Design review of the part built by this model. Coordinates are the model's own, in mm. Face numbers are marked on the shaded views. A direction names the side the tool comes from. Round coordinates to 2 decimals unless told otherwise and drop trailing zeros. Write each loop counter-clockwise with the first axis right and the second up, starting at its lowest first coordinate (ties: lowest second). Pieces come first, ordered by that corner, then holes. Notation, with made-up numbers: (28.25, -38) -> (51.25, -38) arc R14 ccw to (51.25, -16) -> close; hole circle Ø5 at (63.25, 36.25). An arc over 180 degrees is marked (long way). One line per question, with ' | ' between items. Start each with the question number.
1) For probe 1 along Y at (x, z) = (-24.13, -1.2); probe 2 along X at (y, z) = (5.5, 4); probe 3 along Y at (x, z) = (-8.89, -0.9), list the stretches that pass through material, from the lowest coordinate up.
2) For the marked faces 1, 2 and 3, list the 3-axis set-ups (+Z, -Z, +X, -X, +Y, -Y) from which the entire face can be reached by the end or side of a thin tool; tool diameter is ignored.
3) Consider section A-A (z = 2). Give the boundary of the cut face in (x, y).
4) Consider section D-D (x = -24.13). Give the boundary of the cut face in (y, z).
5) Mouldability with a two-part tool opening along X and no side actions: class the marked faces 4, 5, 6 and 7 as +X half, -X half, draft (parallel to the pull), parting line (faces both ways), or undercut.
6) Consider section C-C (y = -15.5). Give the boundary of the cut face in (x, z).
7) Consider section B-B (x = -8.89). Give the boundary of the cut face in (y, z), then the cut area to 3 significant figures.
8) Insertion check: pin 1 Ø3 at (y, z) = (24, 2.5) entering from +X; pin 2 Ø1.3 at (x, z) = (-23.5, 4) entering from -Y; pin 3 Ø0.8 at (x, z) = (-23.5, 6.5) entering from +Y; pin 4 Ø3 at (x, y) = (-24.13, -19.05) entering from +Z. Each pin has a flat end and moves straight along its axis. Give the tip position at first contact, or say it passes through.
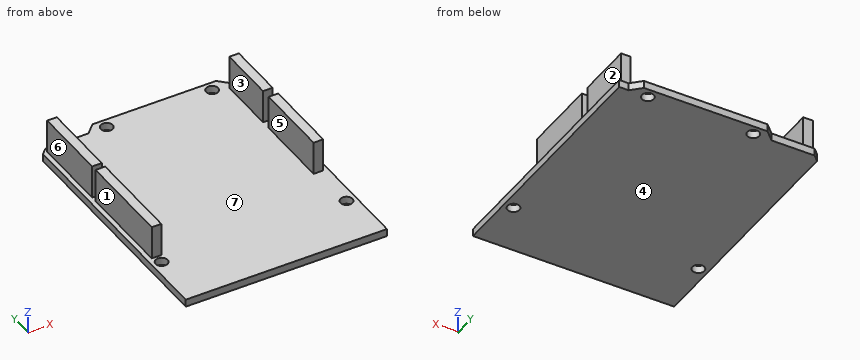
```python
from build123d import *

# Parameters (mm, degrees)
F0_W     = 53.34
F0_H     = 68.58
F1_DEPTH = 2
F3_DEPTH = 2
F6_D     = 3.175
F7_W     = 2.54
F7_H     = 20.32
F7_H_2   = 25.4
F7_H_3   = 15.24
F8_DEPTH = 8.89


# Not quite as in the source:
# - a feature names something its author has since deleted; it is built from what else it names


with BuildPart() as f1:
    # F0 (on Top) → F1 (new body)
    with BuildSketch(Plane.XY):
        Rectangle(F0_W, F0_H)
    extrude(amount=-F1_DEPTH)

    # F2 (on face) → F3 (cut, through all)
    with BuildSketch(Plane.XY):
        Polygon((-25.146, 31.75), (-13.716, 31.75), (-11.176, 34.29), (-26.67, 34.29), (-26.67, 30.226), align=None)
        Polygon((26.67, 34.29), (21.59, 34.29), (24.13, 31.75), (26.67, 31.75), align=None)
    extrude(amount=-F3_DEPTH, mode=Mode.SUBTRACT)

    # F6 (through all)
    with Locations(Plane.XY):
        with Locations((-24.13, -19.05), (24.13, -20.32), (19.05, 31.75), (-8.89, 31.75)):
            Hole(F6_D / 2)

    # F7 (on face) → F8 (join)
    with BuildSketch(Plane.XY):
        with Locations((-24.13, 20.32)):
            Rectangle(F7_W, F7_H)
        with Locations((-24.13, -4.064)):
            Rectangle(F7_W, F7_H_2)
        with Locations((24.13, 22.86)):
            Rectangle(F7_W, F7_H_3)
        with Locations((24.13, 2.54)):
            Rectangle(F7_W, F7_H)
    extrude(amount=F8_DEPTH)


solid = f1.part
```
From the geometry:
1) probe 1: y = -34.29 to -20.64, -17.46 to 31.75 | probe 2: x = -25.4 to -22.86, 22.86 to 25.4 | probe 3: y = -34.29 to 30.16, 33.34 to 34.29
2) face 1: +Z, -X, +Y, -Y | face 2: +Z, +X, +Y, -Y | face 3: +Z, +Y, -Y
3) outline: (-25.4, -16.76) -> (-22.86, -16.76) -> (-22.86, 8.64) -> (-25.4, 8.64) -> close; (-25.4, 10.16) -> (-22.86, 10.16) -> (-22.86, 30.48) -> (-25.4, 30.48) -> close; (22.86, -7.62) -> (25.4, -7.62) -> (25.4, 12.7) -> (22.86, 12.7) -> close; (22.86, 15.24) -> (25.4, 15.24) -> (25.4, 30.48) -> (22.86, 30.48) -> close
4) outline: (-34.29, -2) -> (-20.64, -2) -> (-20.64, 0) -> (-34.29, 0) -> close; (-17.46, -2) -> (31.75, -2) -> (31.75, 0) -> (30.48, 0) -> (30.48, 8.89) -> (10.16, 8.89) -> (10.16, 0) -> (8.64, 0) -> (8.64, 8.89) -> (-16.76, 8.89) -> (-16.76, 0) -> (-17.46, 0) -> close
5) face 4: draft | face 5: undercut | face 6: -X half | face 7: undercut
6) outline: (-26.67, -2) -> (26.67, -2) -> (26.67, 0) -> (-22.86, 0) -> (-22.86, 8.89) -> (-25.4, 8.89) -> (-25.4, 0) -> (-26.67, 0) -> close
7) outline: (-34.29, -2) -> (30.16, -2) -> (30.16, 0) -> (-34.29, 0) -> close; (33.34, -2) -> (34.29, -2) -> (34.29, 0) -> (33.34, 0) -> close | area: 131 mm2
8) pin 1: stops at x = 25.4 | pin 2: stops at y = -16.76 | pin 3: stops at y = 30.48 | pin 4: passes through
